Here's how the part is built. I have some questions about the finished solid (model axes, mm). A direction names the side the tool comes from. Coordinates: 2 decimals unless noted, no trailing zeros. Write each loop counter-clockwise with the first axis right and the second up, starting at its lowest first coordinate (ties: lowest second). Pieces come first, ordered by that corner, then holes.
Item 1: If we section it at B-B (x = -2): Please give me the cut outline in (y, z) (3 decimals), then the cut area to 3 significant figures.
Item 2: For faces 1 (the face through (-76.2, -38, -9)), 2 (the face through (88.9, -38, -3)), 3 (the face through (0, -34.925, 36)), 4 (the face through (0, -76.2, 34)), which set-ups out of +Z, -Z, +X, -X, +Y, -Y let a thin tool reach every point of the face, with its end or its side?
Item 3: If we section it at D-D (y = -49): Please give me the cut outline in (x, z), then the cut area to 3 significant figures.
Item 4: I'm going to push flat-ended pins straight in: pin 1 Ø4 at (x, y) = (85.5, -55.5) entering from +Z; pin 2 Ø1 at (x, y) = (53, -43.5) entering from -Z; pin 3 Ø2 at (x, y) = (73, -34) entering from -Z. Where does each tip first touch, or does it pass through?
Item 5: We'd pull the mould along X, two halves only. Please class faces 5 (the face through (-70.12, -37.57, 16.26)), 6 (the face through (52.99, -38.63, 38.32)), 7 (the face through (-52.93, -38.63, 38.34)): +X half, -X half, draft (parallel to the pull), parting line (faces both ways), or undercut.
Item 6: If I drill on line 1 (X direction, y = -6.5, z = -4.5); line 2 (Z direction, x = -18, y = -30.5); line 3 (X direction, y = -14.5, z = 8), over which ranges is the centre line in solid material (lowest first)?
Item 7: If we section it at C-C (z = 30.5): Please give me the cut outline in (x, y), then the cut area to 3 significant figures.
Item 8: If we section it at A-A (y = -38.1): Please give me the cut outline in (x, z) (3 decimals).
from build123d import *

# Parameters (mm, degrees)
F1_DEPTH = 76.2
F2_R     = 6.35
F4_DEPTH = 50.801


with BuildPart() as f1:
    # F0 (on Front) → F1 (new body)
    with BuildSketch(Plane.XZ):
        Polygon((88.9, -5.741036), (76.2, -5.741036), (76.2, -12.091036), (95.25, -12.091036), (95.25, 3.583144), (53.099017, 38.708964), (-53.099017, 38.708964), (-95.25, 3.583144), (-95.25, -12.091036), (-76.2, -12.091036), (-76.2, -5.741036), (-88.9, -5.741036), (-88.9, 0.608964), (-50.8, 32.358964), (50.8, 32.358964), (88.9, 0.608964), align=None)
    extrude(amount=F1_DEPTH)

    # F2
    f2_edges = [f1.edges().sort_by_distance(p)[0] for p in [
        (-53.099017, -38.1, 38.708964),
        (53.099017, -38.1, 38.708964),
        (95.25, -38.1, 3.583144),
        (95.25, -38.1, -12.091036),
        (-95.25, -38.1, 3.583144),
    ]]
    fillet(f2_edges, radius=F2_R)

    # F3 (on face) → F4 (cut, through all)
    with BuildSketch(Plane.XY.offset(38.708964)):
        with BuildLine():
            Line((25.4, -34.925), (-25.4, -34.925))
            ThreePointArc((-25.4, -34.925), (-28.575, -38.1), (-25.4, -41.275))
            Line((-25.4, -41.275), (25.4, -41.275))
            ThreePointArc((25.4, -41.275), (28.575, -38.1), (25.4, -34.925))
        make_face()
    extrude(amount=-F4_DEPTH, mode=Mode.SUBTRACT)


solid = f1.part
Answer list:
1. outline: (-76.2, 32.359) - (-41.275, 32.359) - (-41.275, 38.709) - (-76.2, 38.709) - close; (-34.925, 32.359) - (0, 32.359) - (0, 38.709) - (-34.925, 38.709) - close
1. area: 444 mm2
2. face 1: -Z, +Y, -Y
2. face 2: +Y, -Y
2. face 3: +Z, -Z
2. face 4: +Z, -Z, +X, -X, -Y
3. outline: (-95.25, -12.09) - (-76.2, -12.09) - (-76.2, -5.74) - (-88.9, -5.74) - (-88.9, 0.61) - (-50.8, 32.36) - (50.8, 32.36) - (88.9, 0.61) - (88.9, -5.74) - (76.2, -5.74) - (76.2, -12.09) - (88.9, -12.09) arc R6.35 ccw to (95.25, -5.74) - (95.25, 0.61) arc R6.35 ccw to (92.97, 5.49) - (54.87, 37.24) arc R6.35 ccw to (50.8, 38.71) - (-50.8, 38.71) arc R6.35 ccw to (-54.87, 37.24) - (-92.97, 5.49) arc R6.35 ccw to (-95.25, 0.61) - close
3. area: 1,650 mm2
4. pin 1: stops at z = 13.37
4. pin 2: stops at z = 30.11
4. pin 3: stops at z = 13.03
5. face 5: undercut
5. face 6: +X half
5. face 7: -X half
6. line 1: x = -95.25 to -88.9, 88.9 to 95.25
6. line 2: z = 32.36 to 38.71
6. line 3: x = -89.95 to -80.03, 80.03 to 89.95
7. outline: (-62.95, -76.2) - (-53.03, -76.2) - (-53.03, 0) - (-62.95, 0) - close; (53.03, -76.2) - (62.95, -76.2) - (62.95, 0) - (53.03, 0) - close
7. area: 1,510 mm2
8. outline: (-95.25, -12.091) - (-76.2, -12.091) - (-76.2, -5.741) - (-88.9, -5.741) - (-88.9, 0.609) - (-50.8, 32.359) - (-28.575, 32.359) - (-28.575, 38.709) - (-50.8, 38.709) arc R6.35 ccw to (-54.865, 37.237) - (-92.965, 5.487) arc R6.35 ccw to (-95.25, 0.609) - close; (28.575, 32.359) - (50.8, 32.359) - (88.9, 0.609) - (88.9, -5.741) - (76.2, -5.741) - (76.2, -12.091) - (88.9, -12.091) arc R6.35 ccw to (95.25, -5.741) - (95.25, 0.609) arc R6.35 ccw to (92.965, 5.487) - (54.865, 37.237) arc R6.35 ccw to (50.8, 38.709) - (28.575, 38.709) - close
